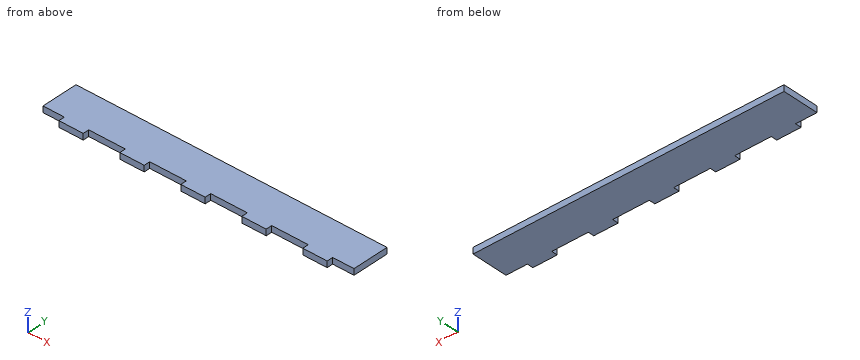
Autodesk Inventor part; units mm, degrees
ref_plane "YZ Plane" through (0, 0, 0) normal (1, 0, 0) x (0, 1, 0)
ref_plane "XZ Plane" through (0, 0, 0) normal (0, 1, 0) x (-1, 0, 0)
ref_plane "XY Plane" through (0, 0, 0) normal (0, 0, 1) x (1, 0, 0)
sketch "Sketch1" plane through (0, 0, 0) normal (0, 0, 1) x (1, 0, 0)
  line L0 (-127.5, 15) -> (127.5, 15)
  line L1 (127.5, 15) -> (127.5, -15)
  line L2 (127.5, -15) -> (-127.5, -15)
  line L3 (-127.5, -15) -> (-127.5, 15)
  line L4 (-127.5, 15) -> (127.5, -15) construction
  line L5 (127.5, 15) -> (-127.5, -15) construction
  point P0 (0, 0)
  dimension "d0" = 255
  dimension "d1" = 30
extrude "Extrusion1" add sketch "Sketch1" along normal blind 5
sketch "Sketch2" plane through (0, 0, 5) normal (0, 0, 1) x (1, 0, 0)
  line L0 (-127.5, -15) -> (127.5, -15)
  line L1 (-110, -15) -> (-90, -15)
  line L2 (-90, -15) -> (-90, -20)
  line L3 (-90, -20) -> (-110, -20)
  line L4 (-110, -20) -> (-110, -15)
  line L5 (-60, -15) -> (-40, -15)
  line L6 (-40, -15) -> (-40, -20)
  line L7 (-40, -20) -> (-60, -20)
  line L8 (-60, -20) -> (-60, -15)
  line L9 (-10, -15) -> (10, -15)
  line L10 (10, -15) -> (10, -20)
  line L11 (10, -20) -> (-10, -20)
  line L12 (-10, -20) -> (-10, -15)
  line L13 (40, -15) -> (60, -15)
  line L14 (60, -15) -> (60, -20)
  line L15 (60, -20) -> (40, -20)
  line L16 (40, -20) -> (40, -15)
  line L17 (90, -15) -> (110, -15)
  line L18 (110, -15) -> (110, -20)
  line L19 (110, -20) -> (90, -20)
  line L20 (90, -20) -> (90, -15)
  point P0 (0, 0)
  point P1 (60, -15)
  point P2 (40, -15)
  point P3 (-90, -15)
  point P4 (-40, -15)
  point P5 (-60, -15)
  point P6 (10, -15)
  point P7 (-10, -15)
  point P8 (110, -15)
  point P9 (90, -15)
  dimension "d4" = 20
  dimension "d5" = 5
  dimension "d6" = 17.5
  dimension "d9" = 50
  dimension "d14" = 17.5
extrude "Extrusion2" add sketch "Sketch2" against normal blind 5
properties part number "Divisória-25cm"
Input: part model. Units: mm. Frame: model coordinates. Round coordinates to 2 decimals unless told otherwise and drop trailing zeros. Loops run counter-clockwise (first coordinate to the right, second up) from the corner with the lowest first, then second, coordinate; pieces in that order, holes last.
1) Section query B-B on x = 28. Return the cut outline in (y, z), plus the area to 3 significant figures.
Ans:
outline: (-15, 0) - (15, 0) - (15, 5) - (-15, 5) - close
area: 150 mm2
2) Section query A-A on z = 1. Return the cut outline in (x, y), plus the area to 3 significant figures.
Ans:
outline: (-127.5, -15) - (-110, -15) - (-110, -20) - (-90, -20) - (-90, -15) - (-60, -15) - (-60, -20) - (-40, -20) - (-40, -15) - (-10, -15) - (-10, -20) - (10, -20) - (10, -15) - (40, -15) - (40, -20) - (60, -20) - (60, -15) - (90, -15) - (90, -20) - (110, -20) - (110, -15) - (127.5, -15) - (127.5, 15) - (-127.5, 15) - close
area: 8,150 mm2
3) Material intervals for line 1 (X direction, y = -17, z = 2.4); line 2 (Y direction, x = -83, z = 1.3), sorted ascending.
Ans:
line 1: x = -110 to -90, -60 to -40, -10 to 10, 40 to 60, 90 to 110
line 2: y = -15 to 15
4) Pin query (flat end, axial travel): pin 1 (2.5 mm diameter, centred on y = -17, z = 1.5, fed in from -X); pin 2 (1.5 mm diameter, centred on x = 122.5, z = 3.5, fed in from -Y); pin 3 (2.5 mm diameter, centred on y = -16.5, z = 1.5, fed in from +X). Return the tip coordinate at first contact, or that it passes through.
Ans:
pin 1: stops at x = -110
pin 2: stops at y = -15
pin 3: stops at x = 110
